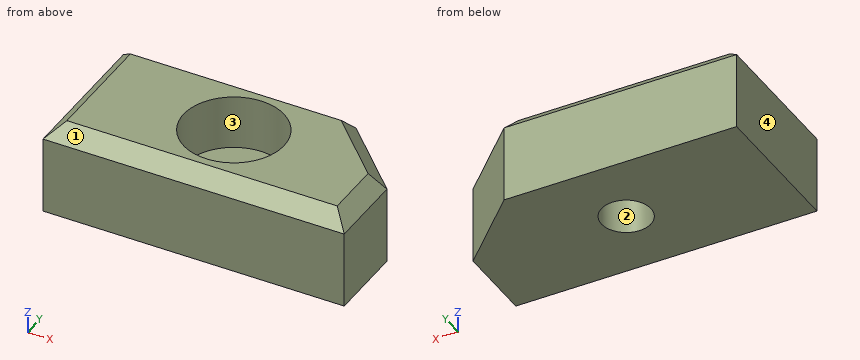
Autodesk Inventor part; units mm, degrees
ref_plane "YZ Plane" through (0, 0, 0) normal (1, 0, 0) x (0, 1, 0)
ref_plane "XZ Plane" through (0, 0, 0) normal (0, 1, 0) x (-1, 0, 0)
ref_plane "XY Plane" through (0, 0, 0) normal (0, 0, 1) x (1, 0, 0)
sketch "Эскиз1" plane through (0, 0, 0) normal (0, 0, 1) x (1, 0, 0)
  line L0 (10, 5) -> (10, -0.4101)
  line L1 (-10, 5) -> (10, 5)
  line L2 (-10, -5) -> (-10, 5)
  line L3 (5.4101, -5) -> (-10, -5)
  line L4 (10, -0.4101) -> (5.4101, -5)
  line L5 (9.75, -0.3065) -> (9.75, 4.75)
  line L6 (9.75, 4.75) -> (-9.75, 4.75)
  line L7 (-9.75, 4.75) -> (-9.75, -4.75)
  line L8 (-9.75, -4.75) -> (5.3065, -4.75)
  line L9 (5.3065, -4.75) -> (9.75, -0.3065)
  circle A0 centre (0, 0) radius 1.6
  line L10 (10, 5) -> (10, -0.4101)
  line L11 (-10, 5) -> (10, 5)
  line L12 (-10, -5) -> (-10, 5)
  line L13 (5.4101, -5) -> (-10, -5)
  line L14 (10, -0.4101) -> (5.4101, -5)
  circle A1 centre (0, 0) radius 1.6
  dimension "d0" = 0.25
extrude "Выдавливание1" add sketch "Эскиз1" along normal blind 6 contours L9 L8 L7 L6 L5
chamfer "Фаска1" distance 1 angle 45 5 edges at (-2.2218, -4.75, 6) (7.5282, -2.5282, 6) (9.75, 2.2218, 6) (0, 4.75, 6) (-9.75, 0, 6)
sketch "Эскиз2" plane through (0, 0, 6) normal (0, 0, 1) x (1, 0, 0)
  circle A0 centre (0, 0) radius 3.25
  dimension "d6" = 6.5
extrude "Выдавливание2" cut sketch "Эскиз2" against normal blind 3.5
mirror "Зеркальное отражение1" about plane through (9.75, 4.75, 0) normal (0, 1, 0) of "Выдавливание1", "Фаска1", "Выдавливание2"
sketch "Эскиз3" plane through (0, 0, 6) normal (0, 0, 1) x (1, 0, 0)
  line L0 (9.75, 4.75) -> (-9.75, 4.75)
  line L1 (-9.75, 4.75) -> (11, 4.75)
  line L2 (11, 4.75) -> (11, -6)
  line L3 (11, -6) -> (-9.75, -6)
  line L4 (-9.75, -6) -> (-9.75, 4.75)
  point P0 (0, 0)
extrude "Выдавливание3" cut sketch "Эскиз3" against normal up to surface (6 mm away)
properties part number "leg3"
The model under review builds one solid part; all positions refer to its coordinate system, in mm. Face numbers are marked on the shaded views. Round coordinates to 2 decimals unless told otherwise and drop trailing zeros. Order: outer loops, then holes, each group sorted by start corner. A loop starts at its lowest first (then second) coordinate and runs counter-clockwise, first axis right, second up.
Item 1: Add section C-C, the plane y = 12.5. State the section outline as (x, z) points.
Working result:
outline: (-9.75, 0) - (7.06, 0) - (7.06, 5) - (5.64, 6) - (1.25, 6) - (1.25, 2.5) - (-1.25, 2.5) - (-1.25, 6) - (-8.75, 6) - (-9.75, 5) - close
Item 2: For pin 1 (5 mm diameter, centred on x = -1, y = 10.5, fed in from +Z); pin 2 (1.5 mm diameter, centred on y = 13, z = 4.5, fed in from +X), all flat-tipped, find the tip position at first contact; note any pin that passes through.
Working result:
pin 1: stops at z = 6
pin 2: stops at x = 7.31
Item 3: Add section D-D, the plane x = -8.5. State the section outline as (y, z) points, and give its area (3 significant figures).
Working result:
outline: (4.75, 0) - (14.25, 0) - (14.25, 5) - (13.25, 6) - (5.75, 6) - (4.75, 5) - close
area: 56.0 mm2
Item 4: Add section A-A, the plane z = 1.5. State the section outline as (x, y) points, and give its area (3 significant figures).
Working result:
outline: (-9.75, 4.75) - (9.75, 4.75) - (9.75, 9.81) - (5.31, 14.25) - (-9.75, 14.25) - close; hole circle Ø3.2 at (0, 9.5)
area: 167 mm2
Item 5: Add section B-B, the plane x = 0. State the section outline as (y, z) points, and give its area (3 significant figures).
Working result:
outline: (4.75, 0) - (7.9, 0) - (7.9, 2.5) - (6.25, 2.5) - (6.25, 6) - (5.75, 6) - (4.75, 5) - close; (11.1, 0) - (14.25, 0) - (14.25, 5) - (13.25, 6) - (12.75, 6) - (12.75, 2.5) - (11.1, 2.5) - close
area: 25.3 mm2
Item 6: Draft analysis for pull direction X (two halves, no side actions). For the marked faces 1, 2, 3 and 4, state which applies: released by +X, released by -X, zero draft, split by the parting line, or undercut.
Working result:
face 1: zero draft
face 2: undercut
face 3: undercut
face 4: released by -X
Item 7: To check wall thickness, follow probe 1 along X at (y, z) = (9.5, 0.95); probe 2 along Y at (x, z) = (0, 4); probe 3 along Y at (x, z) = (0, 1.2). State the ranges of each line that lie inside material, in increasing order.
Working result:
probe 1: x = -9.75 to -1.6, 1.6 to 9.75
probe 2: y = 4.75 to 6.25, 12.75 to 14.25
probe 3: y = 4.75 to 7.9, 11.1 to 14.25
